Build history of the part. All positions in model axes, mm. A direction names the side the tool comes from. Give positions to 0.01 mm unless a question says otherwise; leave off trailing zeros. Order: outer loops, then holes, each group sorted by start corner. A loop starts at its lowest first (then second) coordinate and runs counter-clockwise, first axis right, second up. Notation, with made-up numbers: M 41.5,67.5 L 98.5,67.5 A14 ccw 98.5,86.5 Z; hole C 84,-39.75 d1. An arc over 180 degrees is marked long. One line per item, written item: value.
from build123d import *

# Parameters (mm, degrees)
SKETCH1_W           = 10
SKETCH1_H           = 46
BOSS_EXTRUDE1_DEPTH = 4
LPATTERN2_COUNT     = 4
LPATTERN2_PITCH     = 10


with BuildPart() as part:
    # Sketch1 → Boss-Extrude1 (new body)
    with BuildSketch(Plane.XY):
        Rectangle(SKETCH1_W, SKETCH1_H)
        with BuildLine():
            Line((1.6, 17.5), (1.6, -17.5))
            ThreePointArc((1.6, -17.5), (0, -19.1), (-1.6, -17.5))
            Line((-1.6, -17.5), (-1.6, 17.5))
            ThreePointArc((-1.6, 17.5), (0, 19.1), (1.6, 17.5))
        make_face(mode=Mode.SUBTRACT)
    boss_extrude1 = extrude(amount=BOSS_EXTRUDE1_DEPTH)

    # LPattern2: Boss-Extrude1 ×4
    with Locations(*[(-i * LPATTERN2_PITCH, 0, 0) for i in range(1, LPATTERN2_COUNT)]):
        add(boss_extrude1)


solid = part.part
1) Tool access for faces 4 (the face through (-15, 0, 4)), 5 (the face through (-10, 19.1, 2)): list every direction of +Z, -Z, +X, -X, +Y, -Y with a clear straight run to the whole face (end or side of a thin tool).
Check values:
face 4: +Z, +X, -X, +Y, -Y
face 5: +Z, -Z
2) Saw through at B-B, the plane x = -30. Write the cut outline in (y, z).
Check values:
outline: M -23,0 L -19.1,0 L -19.1,4 L -23,4 Z; M 19.1,0 L 23,0 L 23,4 L 19.1,4 Z
3) Drill centre lines: probe 1 along X at (y, z) = (-2, 0.3); probe 2 along Y at (x, z) = (1, 2.3); probe 3 along Y at (x, z) = (-19.5, 1.6). Where is each one in solid material? Low to high. Write a range as from..to.
Check values:
probe 1: -35..-31.6, -28.4..-21.6, -18.4..-11.6, -8.4..-1.6, 1.6..5
probe 2: -23..-18.75, 18.75..23
probe 3: -23..-19.02, 19.02..23
4) Mould opens along X. For faces 1 (the face through (-30, -19.1, 2)), 2 (the face through (-15, 0, 0)), 3 (the face through (5, 0, 2)) say: released by +X, released by -X, zero draft, split by the parting line, or undercut.
Check values:
face 1: undercut
face 2: zero draft
face 3: released by +X
5) Saw through at A-A, the plane y = 10. Write the cut outline in (x, z).
Check values:
outline: M -35,0 L -31.6,0 L -31.6,4 L -35,4 Z; M -28.4,0 L -21.6,0 L -21.6,4 L -28.4,4 Z; M -18.4,0 L -11.6,0 L -11.6,4 L -18.4,4 Z; M -8.4,0 L -1.6,0 L -1.6,4 L -8.4,4 Z; M 1.6,0 L 5,0 L 5,4 L 1.6,4 Z
6) Saw through at C-C, the plane z = 1.45. Write the cut outline in (x, y).
Check values:
outline: M -35,-23 L 5,-23 L 5,23 L -35,23 Z; hole M -31.6,-17.5 A1.6 ccw -28.4,-17.5 L -28.4,17.5 A1.6 ccw -31.6,17.5 Z; hole M -21.6,-17.5 A1.6 ccw -18.4,-17.5 L -18.4,17.5 A1.6 ccw -21.6,17.5 Z; hole M -11.6,-17.5 A1.6 ccw -8.4,-17.5 L -8.4,17.5 A1.6 ccw -11.6,17.5 Z; hole M -1.6,-17.5 A1.6 ccw 1.6,-17.5 L 1.6,17.5 A1.6 ccw -1.6,17.5 Z
